Check sheet for the modelled part. Datum: model origin and axes. Units: mm. A direction names the side the tool comes from. Give positions to 0.01 mm unless a question says otherwise; leave off trailing zeros. Write each loop counter-clockwise with the first axis right and the second up, starting at its lowest first coordinate (ties: lowest second). Pieces come first, ordered by that corner, then holes. Notation, with made-up numbers: M 0.25,41 L 45.25,41 A3 ccw 45.25,45 Z; hole C -17,58.5 d11. An arc over 180 degrees is marked long. One line per item, written item: value. Start each with the question number.
from build123d import *

# Parameters (mm, degrees)
F0_R     = 15
F1_DEPTH = 30


with BuildPart() as f1:
    # F0 (on Front) → F1 (new body)
    with BuildSketch(Plane.XZ):
        with BuildLine():
            ThreePointArc((-22.716467, 19.594952), (-10.452416, -28.120224), (30, 0))
            ThreePointArc((30, 0), (28.120224, 10.452416), (22.716467, 19.594952))
            ThreePointArc((22.716467, 19.594952), (0, 30), (-22.716467, 19.594952))
        make_face()
        Circle(F0_R, mode=Mode.SUBTRACT)
        with BuildLine():
            ThreePointArc((22.716467, 19.594952), (28.120224, 10.452416), (30, 0))
            ThreePointArc((30, 0), (-10.452416, -28.120224), (-22.716467, 19.594952))
            Line((-22.716467, 19.594952), (-100, -70))
            Line((-100, -70), (100, -70))
            Line((100, -70), (22.716467, 19.594952))
        make_face()
        Polygon((100, -120), (100, -70), (-100, -70), (-100, -120), (-50, -120), (-80, -90), (80, -90), (50, -120), align=None)
    extrude(amount=F1_DEPTH)


solid = f1.part
1) Draft check along X on faces 3 (the flat face through (75, -15, -120)), 4 (the flat face through (-1, -15, -90)), 5 (the flat face through (100, -15, -95)). Enter one of: released by +X, released by -X, zero draft, split by the parting line, or undercut.
2) Tool access check on faces 1 (the flat face through (-60.82, -14.79, -24.58)), 2 (the flat face through (65, -15, -105)). Record the directions out of +Z, -Z, +X, -X, +Y, -Y that give a thin tool (end or side, any length) a straight path to the whole face; none if there is none.
3) Material ranges on L1, parallel to Z at x = 0, y = -7.75; L2, parallel to X at y = -2, z = -111; L3, parallel to X at y = -25.75, z = 1, recorded low to high. Write a range as from..to.
4) Cross-section at D-D (z = -23.5). Record the boundary of the cut face in (x, y).
5) Gauge pin test, flat ends, axial feed: pin 1 (12 mm diameter, centred on x = -72.5, y = -23, fed in from +Z); pin 2 (15 mm diameter, centred on x = 35, y = -14, fed in from -Z); pin 3 (12 mm diameter, centred on y = -10, z = 12, fed in from -X). Record the tip position at first contact, or that the pin passes through.
6) Cross-section at C-C (y = -26). Record the boundary of the cut face in (x, z).
7) Cross-section at A-A (x = 0). Record the boundary of the cut face in (y, z), plus the area to 3 significant figures.
8) Cross-section at B-B (z = -109.5). Record the boundary of the cut face in (x, y).
Data:
1. face 3: zero draft
1. face 4: undercut
1. face 5: released by +X
2. face 1: +Z, -X, +Y, -Y
2. face 2: +Y, -Y
3. L1: z = -90..-15, 15..30
3. L2: x = -100..-59, 59..100
3. L3: x = -38.76..-14.97, 14.97..38.76
4. outline: M -59.89,-30 L 59.89,-30 L 59.89,0 L -59.89,0 Z
5. pin 1: stops at z = -31.16
5. pin 2: stops at z = -90
5. pin 3: stops at x = -34.44
6. outline: M -100,-120 L -50,-120 L -80,-90 L 80,-90 L 50,-120 L 100,-120 L 100,-70 L 22.72,19.59 A30 ccw -22.72,19.59 L -100,-70 Z; hole C 0,0 d30
7. outline: M -30,-90 L 0,-90 L 0,-15 L -30,-15 Z; M -30,15 L 0,15 L 0,30 L -30,30 Z
7. area: 2,700 mm2
8. outline: M -100,-30 L -60.5,-30 L -60.5,0 L -100,0 Z; M 60.5,-30 L 100,-30 L 100,0 L 60.5,0 Z
